Autodesk Inventor part; units mm, degrees
ref_plane "YZ Plane" through (0, 0, 0) normal (1, 0, 0) x (0, 1, 0)
ref_plane "XZ Plane" through (0, 0, 0) normal (0, 1, 0) x (-1, 0, 0)
ref_plane "XY Plane" through (0, 0, 0) normal (0, 0, 1) x (1, 0, 0)
sketch "Sketch1" plane through (0, 0, 0) normal (1, 0, 0) x (0, 1, 0)
  line L0 (2, 0) -> (54, 0)
  line L1 (56, -2) -> (56, -96.5)
  line L2 (54, -98.5) -> (2, -98.5)
  line L3 (0, -96.5) -> (0, -2)
  line L4 (40, -7) -> (32, -7)
  line L5 (30, -9) -> (30, -25)
  line L6 (32, -27) -> (40, -27)
  line L7 (42, -25) -> (42, -9)
  arc A0 (40, -27) -> (42, -25) centre (40, -25) ccw
  arc A1 (32, -7) -> (30, -9) centre (32, -9) ccw
  arc A2 (30, -25) -> (32, -27) centre (32, -25) ccw
  arc A3 (42, -9) -> (40, -7) centre (40, -9) ccw
  line L8 (0, -49.5) -> (56, -49.5)
  line L9 (40, -92) -> (32, -92)
  line L10 (30, -90) -> (30, -74)
  line L11 (32, -72) -> (40, -72)
  line L12 (42, -74) -> (42, -90)
  arc A4 (42, -74) -> (40, -72) centre (40, -74) ccw
  arc A5 (30, -90) -> (32, -92) centre (32, -90) ccw
  arc A6 (32, -72) -> (30, -74) centre (32, -74) ccw
  arc A7 (40, -92) -> (42, -90) centre (40, -90) ccw
  arc A8 (56, -2) -> (54, 0) centre (54, -2) ccw
  arc A9 (54, -98.5) -> (56, -96.5) centre (54, -96.5) ccw
  arc A10 (0, -96.5) -> (2, -98.5) centre (2, -96.5) ccw
  arc A11 (2, 0) -> (0, -2) centre (2, -2) ccw
  point P0 (0, 0)
  point P1 (56, -98.5)
  point P2 (56, 0)
  point P3 (0, -98.5)
  point P4 (42, -7)
  point P5 (30, -27)
  point P6 (42, -27)
  point P7 (42, -92)
  point P8 (30, -72)
  point P9 (42, -72)
  dimension "d0" = 56
  dimension "d1" = 98.5
  dimension "d2" = 7
  dimension "d3" = 30
  dimension "d4" = 12
  dimension "d5" = 20
  dimension "d6" = 2
  dimension "d7" = 49.5
  dimension "d10" = 2
extrude "Extrusion1" add sketch "Sketch1" along normal blind 3
sketch "Boceto2" plane through (3, 0, 0) normal (1, 0, 0) x (0, 0, -1)
  circle A0 centre (43.0768, 43) radius 1.5 construction
  circle A1 centre (55.0768, 43) radius 1.5 construction
  circle A2 centre (43.0768, 33) radius 1.5 construction
  circle A3 centre (55.0768, 33) radius 1.5 construction
  point P0 (0, 0)
hole "SpacersSetHerramientas" at (3, 43, -43.0768) at (3, 33, -43.0768) at (3, 33, -55.0768) at (3, 43, -55.0768) direction (-1, 0, 0) diameter 3 end through all
properties part number "PARED FRONTAL"
Here's how the part is built. I have some questions about the finished solid (model axes, mm). A direction names the side the tool comes from. Round coordinates to 2 decimals unless told otherwise and drop trailing zeros. Loops run counter-clockwise (first coordinate to the right, second up) from the corner with the lowest first, then second, coordinate; pieces in that order, holes last.
1. If we section it at C-C on z = -10.5: Write out the boundary of the cut face in (x, y), plus the area to 3 significant figures.
Answer list:
outline: (0, 0) - (3, 0) - (3, 30) - (0, 30) - close; (0, 42) - (3, 42) - (3, 56) - (0, 56) - close
area: 132 mm2
2. If we section it at A-A on y = 33: Write out the boundary of the cut face in (x, z), plus the area to 4 significant figures.
Answer list:
outline: (0, -98.5) - (3, -98.5) - (3, -92) - (0, -92) - close; (0, -72) - (3, -72) - (3, -56.58) - (0, -56.58) - close; (0, -53.58) - (3, -53.58) - (3, -44.58) - (0, -44.58) - close; (0, -41.58) - (3, -41.58) - (3, -27) - (0, -27) - close; (0, -7) - (3, -7) - (3, 0) - (0, 0) - close
area: 157.5 mm2
3. If we section it at B-B on y = 43: Write out the boundary of the cut face in (x, z), plus the area to 4 significant figures.
Answer list:
outline: (0, -98.5) - (3, -98.5) - (3, -56.58) - (0, -56.58) - close; (0, -53.58) - (3, -53.58) - (3, -44.58) - (0, -44.58) - close; (0, -41.58) - (3, -41.58) - (3, 0) - (0, 0) - close
area: 277.5 mm2
4. If I drill on line 1 along Z through (x, y) = (1.7, 33); line 2 along Y through (x, z) = (0.85, -43); line 3 along Z through (x, y) = (2.25, 39), over which ranges is the centre line in solid material (lowest first)?
Answer list:
line 1: z = -98.5 to -92, -72 to -56.58, -53.58 to -44.58, -41.58 to -27, -7 to 0
line 2: y = 0 to 31.5, 34.5 to 41.5, 44.5 to 56
line 3: z = -98.5 to -92, -72 to -27, -7 to 0
5. Which directions (+Z, -Z, +X, -X, +Y, -Y) give clear straight access to the entire face, cutting with the end or side of a thin tool? Please do faces 1 (the face through (1, 28, 0)), 2 (the face through (1.48, 30.6, -91.43)).
Answer list:
face 1: +Z, +X, -X, +Y, -Y
face 2: +X, -X
6. We'd pull the mould along Y, two halves only. Please class faces 3 (the face through (1, 56, -49)), 4 (the face through (1.479, 33.913, -41.886)), 5 (the face through (1, 28, -98.5)): +Y half, -Y half, draft (parallel to the pull), parting line (faces both ways), or undercut.
Answer list:
face 3: +Y half
face 4: undercut
face 5: draft
7. If we section it at D-D on x = 1.8: Write out the boundary of the cut face in (y, z), plus the area to 3 significant figures.
Answer list:
outline: (0, -96.5) arc R2 ccw to (2, -98.5) - (54, -98.5) arc R2 ccw to (56, -96.5) - (56, -2) arc R2 ccw to (54, 0) - (2, 0) arc R2 ccw to (0, -2) - close; hole (30, -90) arc R2 ccw to (32, -92) - (40, -92) arc R2 ccw to (42, -90) - (42, -74) arc R2 ccw to (40, -72) - (32, -72) arc R2 ccw to (30, -74) - close; hole (30, -25) arc R2 ccw to (32, -27) - (40, -27) arc R2 ccw to (42, -25) - (42, -9) arc R2 ccw to (40, -7) - (32, -7) arc R2 ccw to (30, -9) - close; hole circle Ø3 at (33, -55.08); hole circle Ø3 at (33, -43.08); hole circle Ø3 at (43, -55.08); hole circle Ø3 at (43, -43.08)
area: 5,010 mm2
